The listing builds one solid part. Answer for the finished solid, in the listing's coordinates (mm). Give positions to 0.01 mm unless a question says otherwise; leave off trailing zeros. Order: outer loops, then holes, each group sorted by start corner. A loop starts at its lowest first (then second) coordinate and runs counter-clockwise, first axis right, second up.
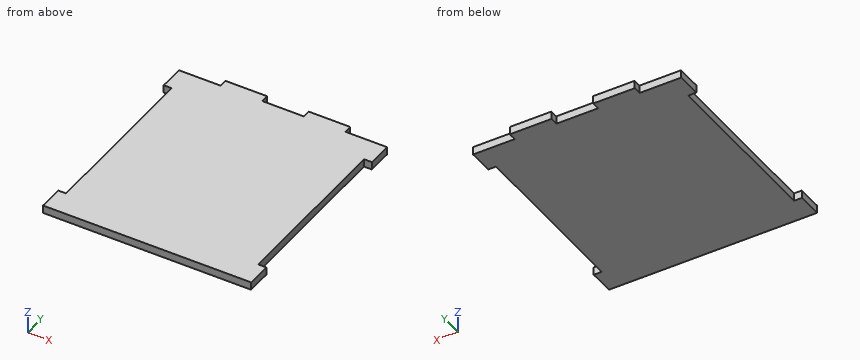
Autodesk Inventor part; units mm, degrees
ref_plane "YZ Plane" through (0, 0, 0) normal (1, 0, 0) x (0, 1, 0)
ref_plane "XZ Plane" through (0, 0, 0) normal (0, 1, 0) x (-1, 0, 0)
ref_plane "XY Plane" through (0, 0, 0) normal (0, 0, 1) x (1, 0, 0)
sketch "Sketch2" plane through (0, 0, 0) normal (0, 0, 1) x (1, 0, 0)
  line L0 (-105, -112.5) -> (105, -112.5)
  line L1 (105, -112.5) -> (105, 112.5)
  line L2 (105, 112.5) -> (-105, 112.5)
  line L3 (-105, 112.5) -> (-105, -112.5)
  line L4 (-105, -112.5) -> (105, 112.5) construction
  line L5 (105, -112.5) -> (-105, 112.5) construction
  point P0 (0, 0)
  dimension "d11" = 225
  dimension "d12" = 210
extrude "Extrusion2" add sketch "Sketch2" along normal blind 8
sketch "Sketch3" plane through (0, 0, 8) normal (0, 0, 1) x (1, 0, 0)
  line L0 (105, 112.5) -> (-105, 112.5)
  line L1 (-63, 112.5) -> (-21, 112.5)
  line L2 (-21, 112.5) -> (-21, 120.5)
  line L3 (-21, 120.5) -> (-63, 120.5)
  line L4 (-63, 120.5) -> (-63, 112.5)
  line L5 (63, 112.5) -> (21, 112.5)
  line L6 (21, 112.5) -> (21, 120.5)
  line L7 (21, 120.5) -> (63, 120.5)
  line L8 (63, 120.5) -> (63, 112.5)
  line L9 (-21, 120.5) -> (21, 120.5) construction
  line L10 (63, 120.5) -> (105, 120.5) construction
  line L11 (-63, 120.5) -> (-105, 120.5) construction
  point P0 (0, 0)
  dimension "d15" = 8
extrude "Extrusion3" add sketch "Sketch3" against normal blind 8
sketch "Sketch4" plane through (0, 0, 8) normal (0, 0, 1) x (1, 0, 0)
  line L0 (-105, 112.5) -> (-105, -112.5)
  line L1 (-105, 87.5) -> (-97, 87.5)
  line L2 (-97, 87.5) -> (-97, -87.5)
  line L3 (-97, -87.5) -> (-105, -87.5)
  line L4 (-105, -87.5) -> (-105, 87.5)
  line L5 (-97, 87.5) -> (-97, 112.5) construction
  line L6 (-97, -87.5) -> (-97, -112.5) construction
  point P0 (0, 0)
  dimension "d20" = 8
  dimension "d21" = 25
extrude "Extrusion4" cut sketch "Sketch4" against normal blind 8
mirror "Mirror2" about plane through (0, 0, 0) normal (1, 0, 0) of "Extrusion4"
properties part number "M06 - Wall Side 1" material "Polycarbonate, Clear"
1) Straight lines are drawn through the part: probe 1 along X at (y, z) = (-43, 4); probe 2 along Y at (x, z) = (-70.5, 4). For each, find the intervals that lie inside material, in ascending order.
Geometry says:
probe 1: x = -97 to 97
probe 2: y = -112.5 to 112.5
2) Given P1, Ø1.5, axis at y = -76.5, z = 1.5, coming from the +X side; P2, Ø4, axis at y = 118, z = 4.5, coming from the +X side; P3, Ø4, axis at y = 18.5, z = 3.5, coming from the -X side, each flat-ended and moving along its own axis, determine where each tip first touches the part or whether it passes through.
Geometry says:
P1: stops at x = 97
P2: stops at x = 63
P3: stops at x = -97
3) Find section A-A (z = 5.75). Write down the section's boundary in (x, y).
Geometry says:
outline: (-105, -112.5) - (105, -112.5) - (105, -87.5) - (97, -87.5) - (97, 87.5) - (105, 87.5) - (105, 112.5) - (63, 112.5) - (63, 120.5) - (21, 120.5) - (21, 112.5) - (-21, 112.5) - (-21, 120.5) - (-63, 120.5) - (-63, 112.5) - (-105, 112.5) - (-105, 87.5) - (-97, 87.5) - (-97, -87.5) - (-105, -87.5) - close
4) Find section C-C (y = -5). Write down the section's boundary in (x, z).
Geometry says:
outline: (-97, 0) - (97, 0) - (97, 8) - (-97, 8) - close
5) Find section B-B (x = 90). Write down the section's boundary in (y, z), then the cut area to 3 significant figures.
Geometry says:
outline: (-112.5, 0) - (112.5, 0) - (112.5, 8) - (-112.5, 8) - close
area: 1,800 mm2
